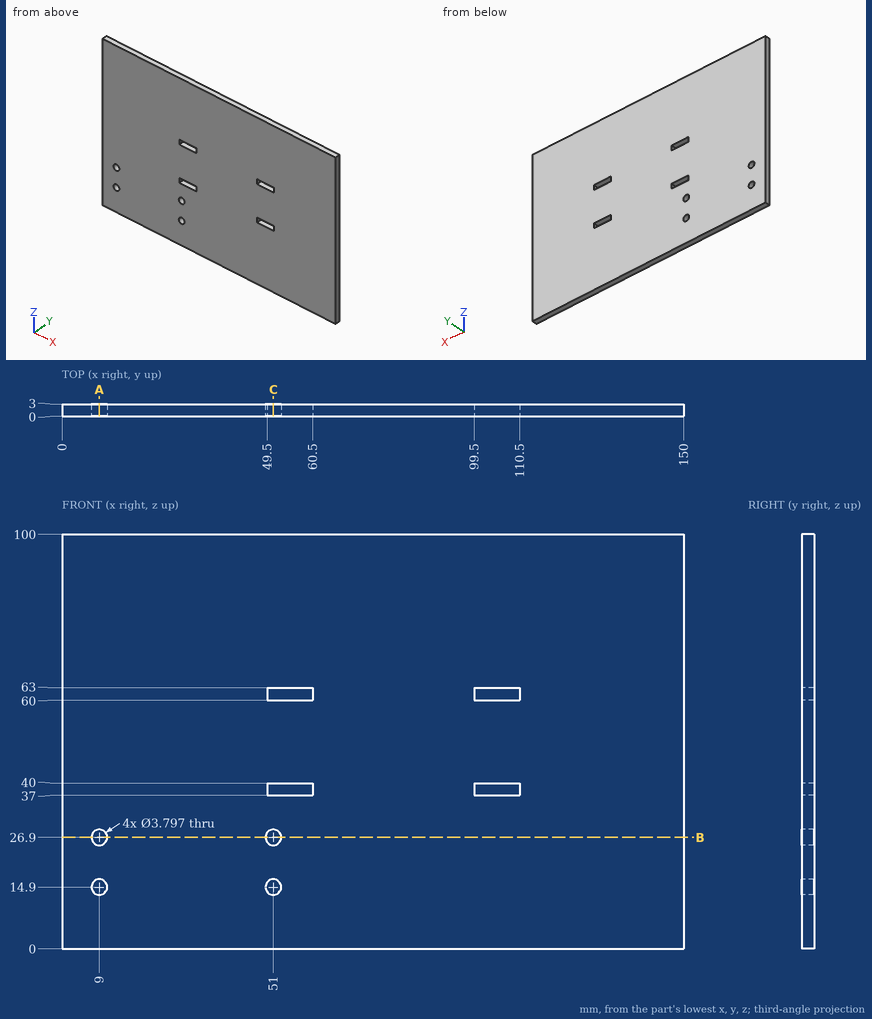
Could you check a few things on this drawing? It's one solid part, dimensions in mm from its lowest x, y, z. Round coordinates to 2 decimals unless told otherwise and drop trailing zeros. Loops run counter-clockwise (first coordinate to the right, second up) from the corner with the lowest first, then second, coordinate; pieces in that order, holes last. Notation, with made-up numbers: M 72.25,19.25 L 112.25,19.25 A16 ccw 112.25,23.25 Z; hole C 64.25,82 d3. An arc over 180 degrees is marked long. Write each question's results on one line, items separated by ' | '. Start each with the question number.
(1) I want a section at B-B (z = 26.9). Please give me the cut outline in (x, y), then the cut area to 3 significant figures.
(2) I want a section at A-A (x = 9). Please give me the cut outline in (y, z).
(3) I want a section at C-C (x = 51). Please give me the cut outline in (y, z), then the cut area to 3 significant figures.
(4) If I drill on probe 1 along Z at (x, y) = (107, 2.6); probe 2 along Z at (x, y) = (51, 2.2); probe 3 along X at (y, z) = (0.95, 14.9), over which ranges is the centre line in solid material (lowest first)? Write a range as from..to.
Solved:
1) outline: M 0,0 L 7.1,0 L 7.1,3 L 0,3 Z; M 10.9,0 L 49.1,0 L 49.1,3 L 10.9,3 Z; M 52.9,0 L 150,0 L 150,3 L 52.9,3 Z | area: 427 mm²
2) outline: M 0,0 L 3,0 L 3,13 L 0,13 Z; M 0,16.8 L 3,16.8 L 3,25 L 0,25 Z; M 0,28.8 L 3,28.8 L 3,100 L 0,100 Z
3) outline: M 0,0 L 3,0 L 3,13 L 0,13 Z; M 0,16.8 L 3,16.8 L 3,25 L 0,25 Z; M 0,28.8 L 3,28.8 L 3,37 L 0,37 Z; M 0,40 L 3,40 L 3,60 L 0,60 Z; M 0,63 L 3,63 L 3,100 L 0,100 Z | area: 259 mm²
4) probe 1: z = 0..37, 40..60, 63..100 | probe 2: z = 0..13, 16.8..25, 28.8..37, 40..60, 63..100 | probe 3: x = 0..7.1, 10.9..49.1, 52.9..150
